```python
from build123d import *

# Parameters (mm, degrees)
F0_R      = 53.975
F1_DEPTH  = 19.05
F2_R      = 29.87
F2_R_2    = 14.63
F3_DEPTH  = 29.21
F5_D      = 6.7564
F6_R      = 53.975
F6_R_2    = 37.846
F7_DEPTH  = 7.62
F8_R      = 12.065
F9_DEPTH  = 29.21
F10_R     = 8.255
F11_DEPTH = 55.881


with BuildPart() as f1:
    # F0 (on Top) → F1 (new body)
    with BuildSketch(Plane.XY):
        Circle(F0_R)
    extrude(amount=F1_DEPTH)

    # F2 (on face) → F3 (join)
    with BuildSketch(Plane.XY.offset(19.05)):
        Circle(F2_R)
        Circle(F2_R_2, mode=Mode.SUBTRACT)
    extrude(amount=F3_DEPTH)

    # F5 (through all)
    with Locations(Plane.XY.offset(48.26)):
        with Locations((0, -22.25), (-22.25, 0), (0, 22.25), (22.25, 0)):
            Hole(F5_D / 2)

    # F6 (on face) → F7 (join)
    with BuildSketch(Plane(origin=(0, 0, 0), x_dir=(1, 0, 0), z_dir=(0, 0, -1))):
        Circle(F6_R)
        Circle(F6_R_2, mode=Mode.SUBTRACT)
    extrude(amount=F7_DEPTH)

    # F8 (on face) → F9 (join, through all)
    with BuildSketch(Plane.XY.offset(19.05)):
        with Locations((13.9193969877, 13.9193969877)):
            Circle(F8_R)
    extrude(amount=F9_DEPTH)

    # F10 (on face) → F11 (cut, through all)
    with BuildSketch(Plane.XY.offset(48.26)):
        with Locations((13.9193969877, 13.9193969877)):
            Circle(F10_R)
    extrude(amount=-F11_DEPTH, mode=Mode.SUBTRACT)


solid = f1.part
```
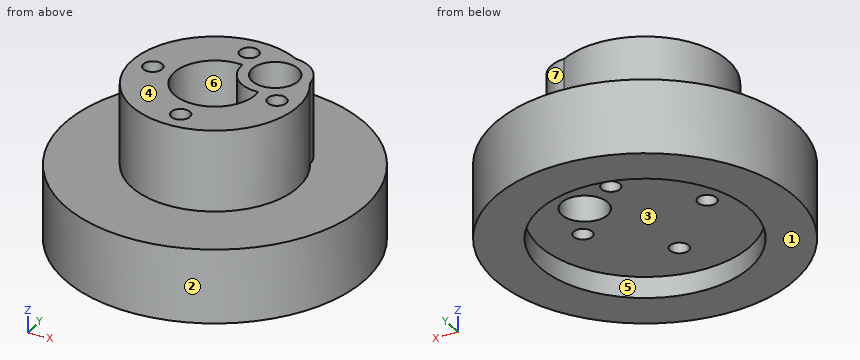
Here's how the part is built. I have some questions about the finished solid (model axes, mm). Face numbers are marked on the shaded views. A direction names the side the tool comes from. Coordinates: 2 decimals unless noted, no trailing zeros. Order: outer loops, then holes, each group sorted by start corner. A loop starts at its lowest first (then second) coordinate and runs counter-clockwise, first axis right, second up. Notation, with made-up numbers: M 47,40 L 54,40 A21 cw 54,45 Z; hole C -28.75,40 d1. An arc over 180 degrees is marked long. Answer as a JSON object with one key per item and string values. Group by question number.
(1) If we mould it in two halves opening along Y, with no side actions, what happens to the marked faces 1, 2 and 3? For each: released by +Y, released by -Y, zero draft, split by the parting line, or undercut.
(2) Suppose I cut it at D-D, the plane z = 12. Please give me the cut outline in (x, y) (3 decimals), then the cut area to 3 significant figures.
(3) For pin 1 (1.5 mm diameter, centred on x = 37.5, z = 19, fed in from -Y); pin 2 (2 mm diameter, centred on x = -10, z = 36, fed in from +Y); pin 3 (10 mm diameter, centred on x = -2, y = -7.5, fed in from +Z), each with a flat end and sliding along its axis, tell me the tip position at first contact or that it passes through.
(4) I need wall thicknesses on probe 1 along Y at (x, z) = (0, 39); probe 2 along Y at (x, z) = (0, 16.5) (3 decimals); probe 3 along X at (y, z) = (0, -3) (3 decimals). Which ranges of each line are inside material? Lowest first, please.
(5) Suppose I cut it at A-A, the plane y = 0. Please give me the cut outline in (x, z) (3 decimals), then the cut area to 3 significant figures.
(6) Suppose I cut it at C-C, the plane y = -22.25. Please give me the cut outline in (x, z).
(7) Which directions (+Z, -Z, +X, -X, +Y, -Y) give clear straight access to the entire face, cutting with the end or side of a thin tool? Please do the marked faces 4, 5, 6 and 7.
Values found:
{
 "1": {"face 1": "zero draft", "face 2": "split by the parting line", "face 3": "undercut"},
 "2": {"outline": "C 0,0 d107.95; hole C -22.25,0 d6.756; hole C 0,-22.25 d6.756; hole C 0,22.25 d6.756; hole C 13.919,13.919 d16.51; hole C 22.25,0 d6.756", "area": "8,790 mm^2"},
 "3": {"pin 1": "stops at y = -39.53", "pin 2": "stops at y = 28.48", "pin 3": "stops at z = 19.05"},
 "4": {"probe 1": "y = -29.87 to -25.63, -18.87 to -14.63, 14.63 to 18.87, 25.63 to 29.87", "probe 2": "y = -53.975 to -25.628, -18.872 to 18.872, 25.628 to 53.975", "probe 3": "x = -53.975 to -37.846, 37.846 to 53.975"},
 "5": {"outline": "M -53.975,-7.62 L -37.846,-7.62 L -37.846,0 L -25.628,0 L -25.628,48.26 L -29.87,48.26 L -29.87,19.05 L -53.975,19.05 Z; M -18.872,0 L 18.872,0 L 18.872,48.26 L 14.63,48.26 L 14.63,19.05 L -14.63,19.05 L -14.63,48.26 L -18.872,48.26 Z; M 25.628,0 L 37.846,0 L 37.846,-7.62 L 53.975,-7.62 L 53.975,19.05 L 29.87,19.05 L 29.87,48.26 L 25.628,48.26 Z", "area": "2,540 mm^2"},
 "6": {"outline": "M -49.18,-7.62 L -30.61,-7.62 L -30.61,0 L -3.38,0 L -3.38,48.26 L -19.93,48.26 L -19.93,19.05 L -49.18,19.05 Z; M 3.38,0 L 30.61,0 L 30.61,-7.62 L 49.18,-7.62 L 49.18,19.05 L 19.93,19.05 L 19.93,48.26 L 3.38,48.26 Z"},
 "7": {"face 4": "+Z, +X, -X, +Y, -Y", "face 5": "-Z", "face 6": "+Z", "face 7": "+Z, +X, +Y"}
}
